Work out the finished part from the listing and answer in its coordinate system (mm). Face numbers are marked on the shaded views. A direction names the side the tool comes from. Round coordinates to 2 decimals unless told otherwise and drop trailing zeros. Order: outer loops, then holes, each group sorted by start corner. A loop starts at its lowest first (then second) coordinate and runs counter-clockwise, first axis right, second up. Notation, with made-up numbers: (32.5, -10.5) - (47.5, -10.5) arc R14 ccw to (47.5, 1.5) - close; hole circle Ø3 at (-12, 18). An arc over 180 degrees is marked (long way). Use one line per item in the form item = value. Start each with the question number.
Q1. The part is cut by section B-B on x = 0. Determine the outline of the cut face in (y, z), plus the area to 3 significant figures.
Q2. The part is cut by section A-A on y = 29.5. Determine the outline of the cut face in (x, z), plus the area to 3 significant figures.
Q3. Given P1, Ø2, axis at x = 8.5, z = 10, coming from the +Y side; P2, Ø1, axis at x = 10.5, z = 13.5, coming from the -Y side; P3, Ø1.5, axis at y = 36, z = 25.5, coming from the +X side, each flat-ended and moving along its own axis, determine where each tip first touches the part or whether it passes through.
Q4. The part is cut by section C-C on z = 7.75. Determine the outline of the cut face in (x, y), plus the area to 3 significant figures.
Q5. The part is cut by section D-D on y = 76.5. Determine the outline of the cut face in (x, z).
Q6. For a pull along X with two mould halves and no side action, classify the marked faces 4, 5 and 6 as +X half, -X half, draft (parallel to the pull), parting line (faces both ways), or undercut.
Q7. Find the intervals of material crossed by line 1 (X direction, y = 5.5, z = 26.75); line 2 (Z direction, x = 30, y = 7); line 3 (Y direction, x = 0, z = 26.6), in increasing order. Write a range as [from, to].
Q8. Which of the six approach directions +Z, -Z, +X, -X, +Y, -Y give full straight-line access (tool end or side, diameter ignored) to the marked faces 1, 2 and 3?
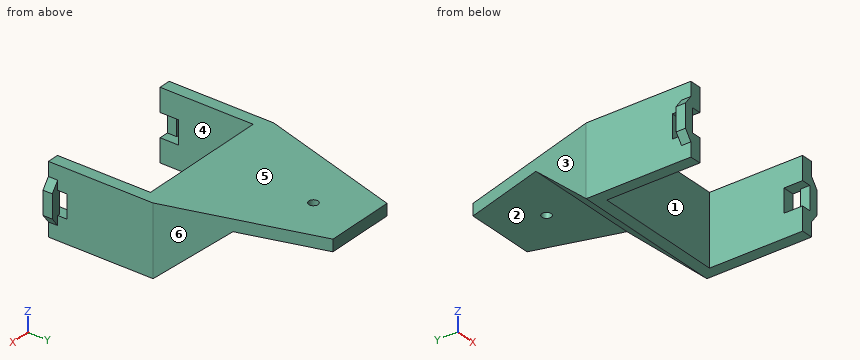
from build123d import *

# Parameters (mm, degrees)
SKETCH_R     = 2
PAD_DEPTH    = 30
SKETCH001_W  = 8
SKETCH001_H  = 10
POCKET_DEPTH = 67.001
PAD001_DEPTH = 4


with BuildPart() as part:
    # Sketch → Pad (new body)
    with BuildSketch(Plane.XY):
        Polygon((-33.5, 0), (-33.5, 45), (-15, 108), (15, 108), (33.5, 45), (33.5, 0), (28.5, 0), (28.5, 40), (-28.5, 40), (-28.5, 0), align=None)
        with Locations((0, 88)):
            Circle(SKETCH_R, mode=Mode.SUBTRACT)
    extrude(amount=PAD_DEPTH)

    # Sketch001 (on Face1 of Pad) → Pocket (cut, through all)
    with BuildSketch(Plane.YZ.offset(33.5)):
        Polygon((45, 0), (73, 25), (108, 25), (108, 0), align=None)
        with Locations((4, 15)):
            Rectangle(SKETCH001_W, SKETCH001_H)
    extrude(amount=-POCKET_DEPTH, mode=Mode.SUBTRACT)

    # Sketch002 (on Face3 of Pocket) → Pad001 (join)
    with BuildSketch(Plane.XZ):
        Polygon((32.5, 20), (33.5, 24), (36.5, 20), (36.5, 10), (33.5, 6), (32.5, 10), align=None)
        Polygon((-32.5, 20), (-33.5, 24), (-36.5, 20), (-36.5, 10), (-33.5, 6), (-32.5, 10), align=None)
    extrude(amount=-PAD001_DEPTH)


solid = part.part
Found:
q1.outline = (40, 0) - (45, 0) - (73, 25) - (86, 25) - (86, 30) - (40, 30) - close; (90, 25) - (108, 25) - (108, 30) - (90, 30) - close
q1.area = 795 mm²
q2.outline = (-33.5, 0) - (-28.5, 0) - (-28.5, 30) - (-33.5, 30) - close; (28.5, 0) - (33.5, 0) - (33.5, 30) - (28.5, 30) - close
q2.area = 300 mm²
q3.P1 = 57.32
q3.P2 = 40
q3.P3 = 33.5
q4.outline = (-34.81, 0) - (-28.5, 0) - (-28.5, 40) - (28.5, 40) - (28.5, 0) - (34.81, 0) - (34.81, 4) - (33.5, 4) - (33.5, 45) - (30.95, 53.68) - (-30.95, 53.68) - (-33.5, 45) - (-33.5, 4) - (-34.81, 4) - close
q4.area = 1,300 mm²
q5.outline = (-24.25, 25) - (24.25, 25) - (24.25, 30) - (-24.25, 30) - close
q6.face_4 = undercut
q6.face_5 = draft
q6.face_6 = +X half
q7.line_1 = [-33.5, -28.5], [28.5, 33.5]
q7.line_2 = [0, 10], [20, 30]
q7.line_3 = [40, 86], [90, 108]
q8.face_1 = +Z, -Z, -Y
q8.face_2 = -Z, +X, -X, +Y
q8.face_3 = +Z, -Z, -X, +Y
